Verification items for the finished model (mm, model axes). A direction names the side the tool comes from. Round coordinates to 2 decimals unless told otherwise and drop trailing zeros. Loops run counter-clockwise (first coordinate to the right, second up) from the corner with the lowest first, then second, coordinate; pieces in that order, holes last. Notation, with made-up numbers: (-29.75, 29) -> (-23.75, 29) arc R13 ccw to (-23.75, 45) -> close; hole circle Ø5 at (-37.5, -5.75). An arc over 180 degrees is marked (long way). Write item = value, one per line.
Autodesk Inventor part; units mm, degrees
ref_plane "YZ Plane" through (0, 0, 0) normal (1, 0, 0) x (0, 1, 0)
ref_plane "XZ Plane" through (0, 0, 0) normal (0, 1, 0) x (-1, 0, 0)
ref_plane "XY Plane" through (0, 0, 0) normal (0, 0, 1) x (1, 0, 0)
ref_plane "Work Plane1" through (0, 0, 0) normal (0, 0, 1) x (1, 0, 0)
sketch "Sketch1" plane through (0, 0, 0) normal (0, 0, 1) x (1, 0, 0)
  line L0 (56.2342, -33.08) -> (-38.85, -33.08)
  line L1 (-38.85, -33.08) -> (-38.85, 33.08)
  line L2 (-38.85, 33.08) -> (56.2342, 33.08)
  line L3 (56.2342, 33.08) -> (56.2342, -33.08)
  line L4 (-32.5, 25) -> (-32.5, -25)
  line L5 (49.4242, -28) -> (-29.5, -28)
  line L6 (52.4242, 25) -> (52.4242, -25)
  line L7 (49.4242, 28) -> (-29.5, 28)
  line L8 (-34.405, 29.905) -> (54.3292, 29.905)
  line L9 (54.3292, 29.905) -> (54.3292, -29.905)
  line L10 (54.3292, -29.905) -> (-34.405, -29.905)
  line L11 (-34.405, -29.905) -> (-34.405, 29.905)
  line L12 (-36.31, 30.54) -> (53.6942, 30.54)
  line L13 (53.6942, 30.54) -> (53.6942, -30.54)
  line L14 (53.6942, -30.54) -> (-36.31, -30.54)
  line L15 (-36.31, -30.54) -> (-36.31, 30.54)
  point P0 (0, 0)
  dimension "d18" = 2.54
  dimension "d19" = 2.54
  dimension "d20" = 2.54
  dimension "d27" = 0.635
  dimension "d28" = 2.54
  dimension "d30" = 3.81
  dimension "d31" = 3.81
  dimension "d33" = 2.54
extrude "Extrusion1" add sketch "Sketch1" along normal blind 25.4 contours L0 L1 L2 L3 | L11 L10 L13 L14 L15 L12 L8
fillet "Fillet1" radius 3.175 4 edges at (-38.85, 33.08, 12.7) (-38.85, -33.08, 12.7) (56.2342, -33.08, 12.7) (56.2342, 33.08, 12.7)
sketch "Sketch3" plane through (56.2342, -29.905, 0) normal (1, 0, 0) x (0, 0, -1)
  line L0 (-20.459, 4.3043) -> (-20.459, 20.1843)
  line L1 (-6.959, 4.3043) -> (-20.459, 4.3043)
  line L2 (-6.959, 20.1843) -> (-20.459, 20.1843)
  line L3 (-6.959, 4.3043) -> (-6.959, 20.1843)
  line L4 (-22.449, 27.9943) -> (-22.449, 33.9943)
  line L5 (-13.7386, 23.4443) -> (-16.7386, 23.4443)
  line L6 (-16.7386, 38.5443) -> (-13.7386, 38.5443)
  line L7 (-16.7386, 38.5443) -> (-13.7386, 38.5443)
  line L8 (-7.829, 30.9743) -> (-7.829, 27.9943)
  line L9 (-23.084, 22.8093) -> (-7.194, 22.8093)
  line L10 (-7.194, 22.8093) -> (-7.194, 39.1793)
  line L11 (-7.194, 39.1793) -> (-23.084, 39.1793)
  line L12 (-23.084, 39.1793) -> (-23.084, 22.8093)
  line L13 (-20.84, 3.9233) -> (-6.578, 3.9233)
  line L14 (-6.578, 3.9233) -> (-6.578, 20.5653)
  line L15 (-6.578, 20.5653) -> (-20.84, 20.5653)
  line L16 (-20.84, 20.5653) -> (-20.84, 3.9233)
  point P0 (0, 29.905)
  dimension "d9" = 0.635
  dimension "d10" = 0.635
  dimension "d11" = 0.635
  dimension "d12" = 0.635
  dimension "d13" = 0.381
  dimension "d14" = 0.381
  dimension "d15" = 0.381
  dimension "d16" = 0.381
extrude "Extrusion2" cut sketch "Sketch3" against normal up to surface (1.905 mm away) contours L0 L2 L3 L1 | L12 L11 L10 L9 | L16 L15 L14 L13
sketch "Sketch4" plane through (0, 0, 25.4) normal (0, 0, 1) x (1, 0, 0)
  line L0 (-38.85, 29.905) -> (-38.85, -29.905)
  arc A0 (56.2342, 29.905) -> (53.0592, 33.08) centre (53.0592, 29.905) ccw
  line L1 (53.0592, 33.08) -> (-35.675, 33.08)
  arc A1 (-35.675, 33.08) -> (-38.85, 29.905) centre (-35.675, 29.905) ccw
  line L2 (-38.85, 29.905) -> (-38.85, -29.905)
  arc A2 (-38.85, -29.905) -> (-35.675, -33.08) centre (-35.675, -29.905) ccw
  line L3 (-35.675, -33.08) -> (53.0592, -33.08)
  arc A3 (53.0592, -33.08) -> (56.2342, -29.905) centre (53.0592, -29.905) ccw
  line L4 (56.2342, -29.905) -> (56.2342, 29.905)
  line L5 (-34.405, 29.905) -> (54.3292, 29.905)
  line L6 (54.3292, 29.905) -> (54.3292, -29.905)
  line L7 (54.3292, -29.905) -> (-34.405, -29.905)
  line L8 (-34.405, -29.905) -> (-34.405, 29.905)
  point P0 (0, 0)
extrude "Extrusion3" add sketch "Sketch4" along normal blind 2.54 contours A1 L1 A0 L4 A3 L3 A2 L0 | L5 L6 L7 L8
ref_plane "Work Plane2" through (0, 0, 0) normal (0, 0, 1) x (1, 0, 0)
sketch "Sketch5" plane through (0, 0, 0) normal (0, 0, 1) x (1, 0, 0)
  line L0 (53.0592, 33.08) -> (-35.675, 33.08)
  line L1 (-35.675, 33.08) -> (-35.675, 39.43)
  line L2 (-25.515, 33.08) -> (-25.515, 39.43)
  arc A0 (-25.515, 39.43) -> (-35.675, 39.43) centre (-30.595, 39.43) ccw
  line L3 (-35.675, 33.08) -> (-25.515, 33.08)
  line L4 (8.6921, 33.08) -> (8.6921, -33.08)
  line L5 (-35.675, -33.08) -> (53.0592, -33.08)
  line L6 (-38.85, 29.905) -> (-38.85, -29.905)
  line L7 (-38.85, 0) -> (57.3991, 0)
  line L8 (53.0592, 33.08) -> (53.0592, 39.43)
  line L9 (42.8992, 33.08) -> (42.8992, 39.43)
  arc A1 (53.0592, 39.43) -> (42.8992, 39.43) centre (47.9792, 39.43) ccw
  line L10 (53.0592, 33.08) -> (42.8992, 33.08)
  line L11 (53.0592, -33.08) -> (-35.675, -33.08)
  line L12 (-35.675, -33.08) -> (-35.675, -39.43)
  line L13 (-25.515, -33.08) -> (-25.515, -39.43)
  arc A2 (-35.675, -39.43) -> (-25.515, -39.43) centre (-30.595, -39.43) ccw
  line L14 (-35.675, -33.08) -> (-25.515, -33.08)
  line L15 (42.8992, -33.08) -> (42.8992, -39.43)
  line L16 (53.0592, -33.08) -> (53.0592, -39.43)
  arc A3 (42.8992, -39.43) -> (53.0592, -39.43) centre (47.9792, -39.43) ccw
  point P0 (0, 0)
  point P1 (42.8992, 33.08)
  point P2 (42.8992, -33.08)
  point P3 (-25.515, -33.08)
  dimension "d34" = 6.35
  dimension "d35" = 10.16
extrude "Extrusion4" add sketch "Sketch5" along normal blind 2.54
properties part number "RPi Case"
(1) Go/stop test with flat-tipped pins: pin 1 Ø8.5 at (x, z) = (17.5, 9.5) entering from +Y; pin 2 Ø3 at (x, y) = (45.5, -36.5) entering from +Z; pin 3 Ø4 at (y, z) = (6, 18) entering from +X (3 decimals). Record where each tip stops, or that it passes through.
Filled sheet:
pin_1 = 33.08
pin_2 = 2.54
pin_3 = -34.405
(2) Sectioned sample at C-C, the plane x = 13.5. Record the cut outline in (y, z) (3 decimals).
Filled sheet:
outline = (-33.08, 0) -> (-29.905, 0) -> (-29.905, 25.4) -> (29.905, 25.4) -> (29.905, 0) -> (33.08, 0) -> (33.08, 27.94) -> (-33.08, 27.94) -> close
(3) Set-up check for faces 1 (the face through (-35.675, 36, 1)), 2 (the face through (54.329, 0, 7)), 3 (the face through (42.899, 36, 1)), 4 (the face through (-31, 39, 2.54)): record each of +Z, -Z, +X, -X, +Y, -Y from which the full face is reachable in a straight line by a thin tool's end or side.
Filled sheet:
face_1 = +Z, -Z, -X, +Y
face_2 = -Z
face_3 = +Z, -Z, +Y
face_4 = +Z, +X, -X, +Y
(4) Draft check along Y on faces 5 (the face through (9, 29.905, 13)), 6 (the face through (55.329, 32.125, 14.166)), 7 (the face through (-31, -39, 2.54)). Enter one of: released by +Y, released by -Y, zero draft, split by the parting line, or undercut.
Filled sheet:
face_5 = undercut
face_6 = released by +Y
face_7 = zero draft
(5) Sectioned sample at B-B, the plane z = 4.5. Record the cut outline in (x, y) (3 decimals).
Filled sheet:
outline = (-38.85, -29.905) arc R3.175 ccw to (-35.675, -33.08) -> (53.059, -33.08) arc R3.175 ccw to (56.234, -29.905) -> (56.234, 29.905) arc R3.175 ccw to (53.059, 33.08) -> (-35.675, 33.08) arc R3.175 ccw to (-38.85, 29.905) -> close; hole (-34.405, -29.905) -> (54.329, -29.905) -> (54.329, 29.905) -> (-34.405, 29.905) -> close
(6) Sectioned sample at A-A, the plane y = -23.5. Record the cut outline in (x, z) (3 decimals), and give its area (3 significant figures).
Filled sheet:
outline = (-38.85, 0) -> (-34.405, 0) -> (-34.405, 25.4) -> (54.329, 25.4) -> (54.329, 20.84) -> (56.234, 20.84) -> (56.234, 27.94) -> (-38.85, 27.94) -> close; (54.329, 0) -> (56.234, 0) -> (56.234, 6.578) -> (54.329, 6.578) -> close
area = 376 mm2
(7) Sectioned sample at D-D, the plane z = 19.5. Record the cut outline in (x, y) (3 decimals).
Filled sheet:
outline = (-38.85, -29.905) arc R3.175 ccw to (-35.675, -33.08) -> (53.059, -33.08) arc R3.175 ccw to (56.234, -29.905) -> (56.234, -25.982) -> (54.329, -25.982) -> (54.329, -29.905) -> (-34.405, -29.905) -> (-34.405, 29.905) -> (54.329, 29.905) -> (54.329, 9.274) -> (56.234, 9.274) -> (56.234, 29.905) arc R3.175 ccw to (53.059, 33.08) -> (-35.675, 33.08) arc R3.175 ccw to (-38.85, 29.905) -> close; (54.329, -9.34) -> (56.234, -9.34) -> (56.234, -7.096) -> (54.329, -7.096) -> close
(8) Material ranges on probe 1 along X at (y, z) = (-13.5, 2.5) (3 decimals); probe 2 along Y at (x, z) = (37.5, 11) (3 decimals); probe 3 along Z at (x, y) = (19, -3), recorded low to high. Write a range as from..to.
Filled sheet:
probe_1 = -38.85..-34.405, 54.329..56.234
probe_2 = -33.08..-29.905, 29.905..33.08
probe_3 = 25.4..27.94
